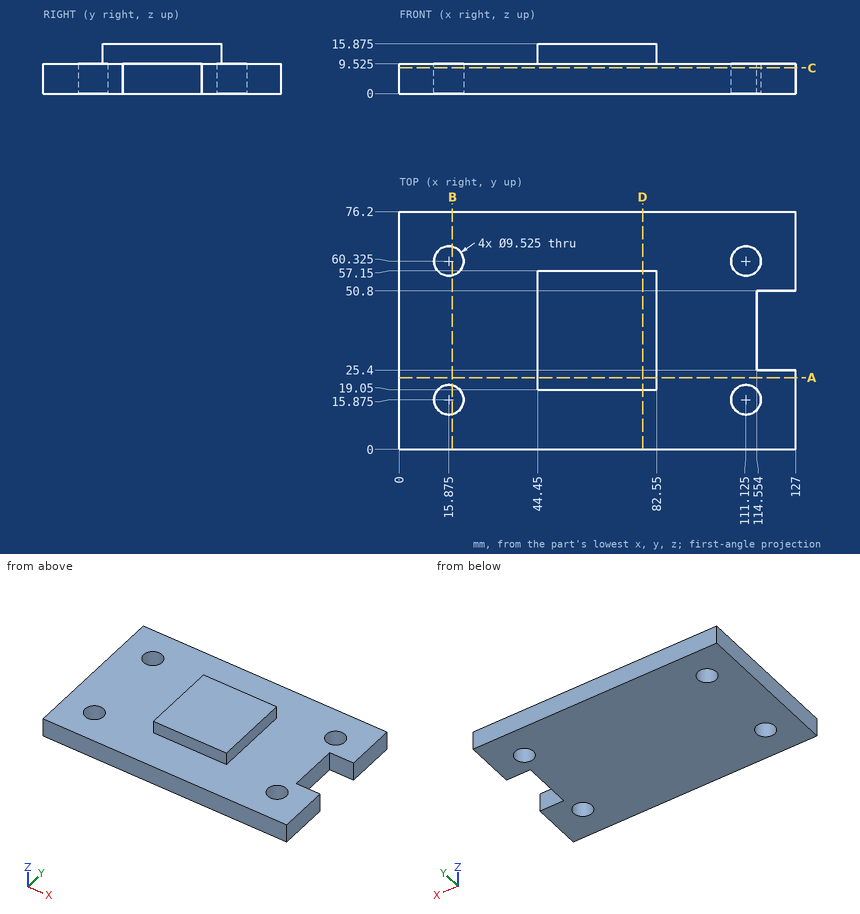
Print and shaded views of the part. All mm, measured from the part's lowest x, y and z. Give positions to 0.01 mm unless a question says otherwise; leave off trailing zeros. Write each loop counter-clockwise with the first axis right and the second up, starting at its lowest first coordinate (ties: lowest second). Pieces come first, ordered by that corner, then holes. Notation, with made-up numbers: (-26.5, -29.75) - (29.5, -29.75) arc R14 ccw to (29.5, -9.75) - close; hole circle Ø4 at (-5.5, 13). An arc over 180 degrees is marked (long way). Put each result on its own line as item: value.
(1) Saw through at B-B (x = 17). List the corners of the cut face in (y, z) (3 decimals), then the cut area to 3 significant figures.
Working result:
outline: (0, 0) - (11.247, 0) - (11.247, 9.525) - (0, 9.525) - close; (20.503, 0) - (55.697, 0) - (55.697, 9.525) - (20.503, 9.525) - close; (64.953, 0) - (76.2, 0) - (76.2, 9.525) - (64.953, 9.525) - close
area: 549 mm^2
(2) Wall check: L1, parallel to Z at x = 75, y = 8 (3 decimals); L2, parallel to X at y = 15, z = 5.25; L3, parallel to X at y = 23, z = 9.75. Give the ranges that are in metal, low to high.
Working result:
L1: 0 to 9.525
L2: 0 to 11.19, 20.56 to 106.44, 115.81 to 127
L3: 44.45 to 82.55
(3) Drop flat-ended pins along their axis: pin 1 Ø7.5 at (y, z) = (37.5, 5) entering from +X; pin 2 Ø2 at (x, y) = (36.5, 46.5) entering from +Z (3 decimals); pin 3 Ø1.9 at (y, z) = (35.5, 13) entering from -X. Give the stop position or say it passes through.
Working result:
pin 1: x = 114.55
pin 2: z = 9.525
pin 3: x = 44.45
(4) Saw through at A-A (y = 23). List the corners of the cut face in (x, z) (3 decimals), then the cut area to 3 significant figures.
Working result:
outline: (0, 0) - (127, 0) - (127, 9.525) - (82.55, 9.525) - (82.55, 15.875) - (44.45, 15.875) - (44.45, 9.525) - (0, 9.525) - close
area: 1,450 mm^2
(5) Saw through at C-C (z = 8.25). List the corners of the cut face in (x, y) (1 decimal), then the cut area to 3 significant figures.
Working result:
outline: (0, 0) - (127, 0) - (127, 25.4) - (114.6, 25.4) - (114.6, 50.8) - (127, 50.8) - (127, 76.2) - (0, 76.2) - close; hole circle Ø9.5 at (15.9, 15.9); hole circle Ø9.5 at (15.9, 60.3); hole circle Ø9.5 at (111.1, 15.9); hole circle Ø9.5 at (111.1, 60.3)
area: 9,080 mm^2
(6) Saw through at D-D (x = 78). List the corners of the cut face in (y, z) (3 decimals).
Working result:
outline: (0, 0) - (76.2, 0) - (76.2, 9.525) - (57.15, 9.525) - (57.15, 15.875) - (19.05, 15.875) - (19.05, 9.525) - (0, 9.525) - close
